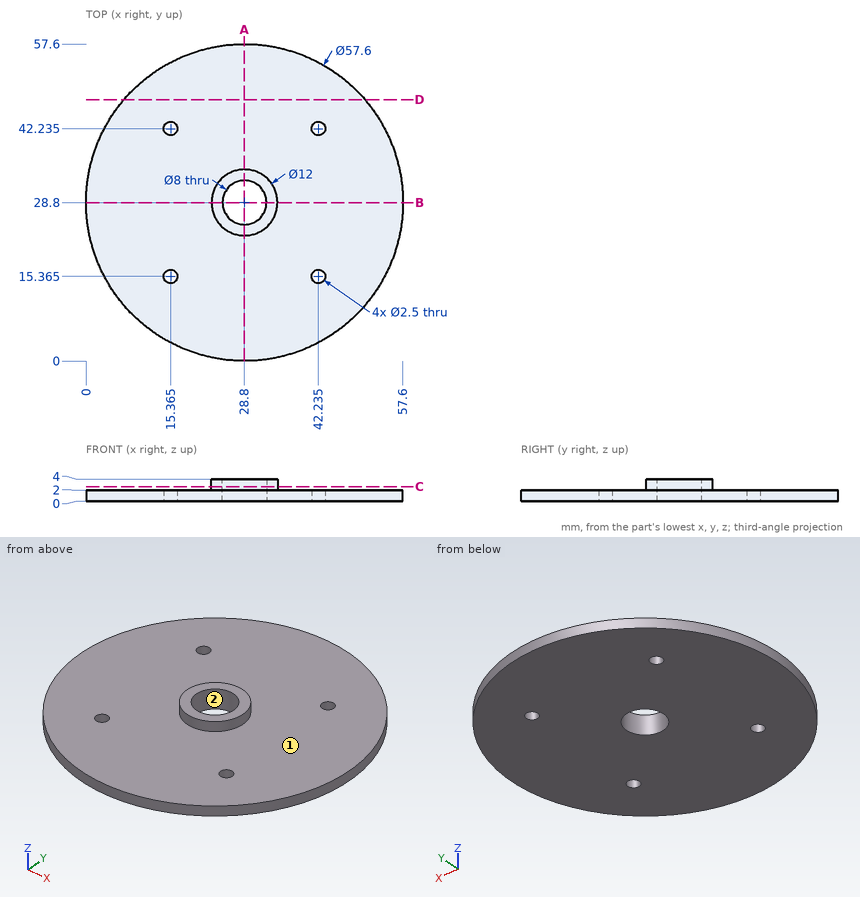
Geometry check sheet. Reference: drawing and pictorial views, mm from the part's lowest x, y, z. Round coordinates to 2 decimals unless told otherwise and drop trailing zeros. Write each loop counter-clockwise with the first axis right and the second up, starting at its lowest first coordinate (ties: lowest second). Pieces come first, ordered by that corner, then holes.
Item 1: Mould release check, pull along Y, two halves, no side actions. Record for the marked faces 1 and 2: +Y half, -Y half, draft (parallel to the pull), parting line (faces both ways), or undercut.
Determined:
face 1: draft
face 2: undercut
Item 2: Material ranges on line 1 along Y through (x, z) = (28.8, 2.9); line 2 along Y through (x, z) = (28.8, 0.9); line 3 along X through (y, z) = (29, 0.95) (3 decimals), recorded low to high.
Determined:
line 1: y = 22.8 to 24.8, 32.8 to 34.8
line 2: y = 0 to 24.8, 32.8 to 57.6
line 3: x = 0.001 to 24.805, 32.795 to 57.599
Item 3: Section check A-A (x = 28.8). Record the boundary of the cut face in (y, z), plus the area to 3 significant figures.
Determined:
outline: (0, 0) - (24.8, 0) - (24.8, 4) - (22.8, 4) - (22.8, 2) - (0, 2) - close; (32.8, 0) - (57.6, 0) - (57.6, 2) - (34.8, 2) - (34.8, 4) - (32.8, 4) - close
area: 107 mm2
Item 4: Section check D-D (y = 47.5). Record the boundary of the cut face in (x, z).
Determined:
outline: (6.9, 0) - (50.7, 0) - (50.7, 2) - (6.9, 2) - close
Item 5: Section check C-C (z = 2.6). Record the boundary of the cut face in (x, y), plus the area to 3 significant figures.
Determined:
outline: circle Ø12 at (28.8, 28.8); hole circle Ø8 at (28.8, 28.8)
area: 62.8 mm2
Item 6: Go/stop test with flat-tipped pins: pin 1 Ø5 at (x, y) = (45.5, 26) entering from +Z; pin 2 Ø1 at (x, z) = (49.5, 1) entering from -Y; pin 3 Ø7 at (x, y) = (28.8, 28.8) entering from -Z. Record where each tip stops, or that it passes through.
Determined:
pin 1: stops at z = 2
pin 2: stops at y = 8.27
pin 3: passes through
